from build123d import *

# Parameters (mm, degrees)
SKETCH1_R           = 5.588
SKETCH1_R_2         = 4.572
BOSS_EXTRUDE1_DEPTH = 12.7
SKETCH3_R           = 1.5875
BOSS_EXTRUDE3_DEPTH = 1.5875
SKETCH6_OUTSIDE_W   = 19.008
SKETCH6_OUTSIDE_H   = 19.008
SKETCH6_OUTSIDE_R   = 4.191
CUT_EXTRUDE4_DEPTH  = 25.4


with BuildPart() as part:
    # Sketch1 → Boss-Extrude1 (new body)
    with BuildSketch(Plane(origin=(0, 0, 0), x_dir=(1, 0, 0), z_dir=(0, 1, 0))):
        Circle(SKETCH1_R)
        Circle(SKETCH1_R_2, mode=Mode.SUBTRACT)
    extrude(amount=BOSS_EXTRUDE1_DEPTH)

    # Sketch2 → Revolve2 (revolve)
    with BuildSketch(Plane.XY):
        Polygon((-5.588, 12.7), (-4.572, 12.7), (-2.159, 15.113), (0, 15.113), (0, 17.145), (-2.159, 17.145), (-4.191, 17.145), align=None)
    revolve(axis=Axis((0, 15.113, 0), (0, 1, 0)))

    # Sketch3 → Boss-Extrude3 (add, symmetric)
    with BuildSketch(Plane.XY):
        with BuildLine():
            Line((-4.191, 17.145), (4.191, 17.145))
            Line((4.191, 17.145), (4.191, 20.32))
            ThreePointArc((4.191, 20.32), (0, 24.511), (-4.191, 20.32))
            Line((-4.191, 20.32), (-4.191, 17.145))
        make_face()
        with Locations((0, 20.32)):
            Circle(SKETCH3_R, mode=Mode.SUBTRACT)
    extrude(amount=BOSS_EXTRUDE3_DEPTH, both=True)

    # Sketch6 outside → Cut-Extrude4 (cut)
    with BuildSketch(Plane.XZ.offset(-17.145)):
        Rectangle(SKETCH6_OUTSIDE_W, SKETCH6_OUTSIDE_H)
        Circle(SKETCH6_OUTSIDE_R, mode=Mode.SUBTRACT)
    extrude(amount=-CUT_EXTRUDE4_DEPTH, mode=Mode.SUBTRACT)


solid = part.part
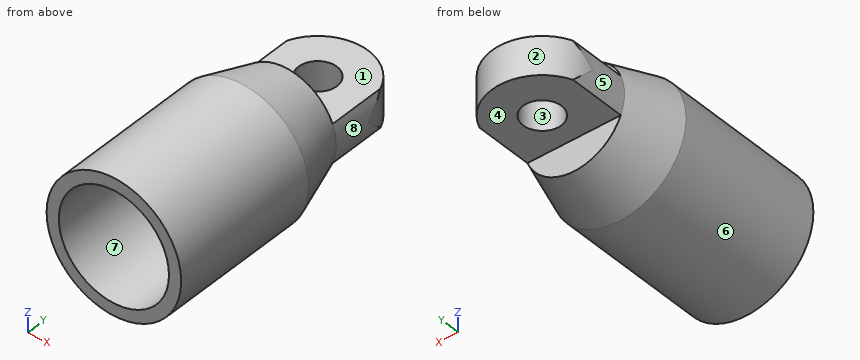
Source: CAD feature listing. Evaluate the final solid. Frame: model axes, mm. Face numbers are marked on the shaded views. A direction names the side the tool comes from. Round coordinates to 2 decimals unless told otherwise and drop trailing zeros. Write each loop counter-clockwise with the first axis right and the second up, starting at its lowest first coordinate (ties: lowest second). Pieces come first, ordered by that corner, then holes. Notation, with made-up numbers: M 23.5,34.25 L 36.5,34.25 A6 cw 36.5,44.25 Z; hole C 61,45 d7. An arc over 180 degrees is marked long. One line per item, written item: value. Start each with the question number.
Item 1: Section query A-A (y = 19.25). Return the cut outline in (x, z).
Item 2: Ray query, L1, parallel to Z at x = 0, y = 3.25; L2, parallel to Y at x = 0, z = -0.55. Return the intervals inside material, ascending. Write a range as from..to.
Item 3: Mould query, pull axis Y, two halves, no side actions, for the marked faces 1, 2 and 3. Classes: pulls with the +Y half, pulls with the -Y half, needs draft (parallel to the pull), parting line crosses it, or undercut.
Item 4: Set-up query: the marked faces 4, 5, 6, 7 and 8. Return all of +Z, -Z, +X, -X, +Y, -Y with unobstructed straight access to the full face (end or side cutting, diameter ignored); none if empty.
Item 5: Pin query (flat end, axial travel): pin 1 (1 mm diameter, centred on x = 2.5, z = -2, fed in from -Y); pin 2 (0.8 mm diameter, centred on x = 2, z = 3, fed in from +Y) (3 decimals); pin 3 (1.3 mm diameter, centred on x = 0, z = -0.5, fed in from -Y). Return the tip coordinate at first contact, or that it passes through.
Item 6: Section query B-B (x = 0). Return the cut outline in (y, z) (1 decimal).
Item 7: Section query C-C (y = 2). Return the cut outline in (x, z).
Result set:
1. outline: M -3.88,-1.59 L -1.17,-1.59 L -1.17,1.59 L -3.88,1.59 A4.19 ccw Z; M 1.17,-1.59 L 3.88,-1.59 A4.19 ccw 3.88,1.59 L 1.17,1.59 Z
2. L1: z = -5.59..-4.57, 4.57..5.59
2. L2: y = 15.11..18.73, 21.91..24.51
3. face 1: needs draft
3. face 2: pulls with the +Y half
3. face 3: undercut
4. face 4: -Z, +X, -X, +Y
4. face 5: -X, +Y
4. face 6: +Y, -Y
4. face 7: -Y
4. face 8: +X, +Y
5. pin 1: stops at y = 13.57
5. pin 2: stops at y = 17.145
5. pin 3: stops at y = 15.11
6. outline: M 0,-5.6 L 12.7,-5.6 L 17.1,-4.2 L 17.1,-1.6 L 18.7,-1.6 L 18.7,1.6 L 17.1,1.6 L 17.1,4.2 L 12.7,5.6 L 0,5.6 L 0,4.6 L 12.7,4.6 L 15.1,2.2 L 15.1,-2.2 L 12.7,-4.6 L 0,-4.6 Z; M 21.9,-1.6 L 24.5,-1.6 L 24.5,1.6 L 21.9,1.6 Z
7. outline: C 0,0 d11.18; hole C 0,0 d9.14
